Here's how the part is built. I have some questions about the finished solid (model axes, mm). Coordinates: 2 decimals unless noted, no trailing zeros. Write each loop counter-clockwise with the first axis right and the second up, starting at its lowest first coordinate (ties: lowest second). Pieces come first, ordered by that corner, then holes.
Item 1: If I drill on line 1 (X direction, y = -156, z = 2.75); line 2 (Y direction, x = -67.5, z = -1.75), over which ranges is the centre line in solid material (lowest first)?
Item 2: I'm going to push flat-ended pins straight in: pin 1 Ø10.5 at (x, y) = (-156, -156) entering from -Z; pin 2 Ø2.5 at (x, z) = (9, -1) entering from -Y; pin 3 Ø1.5 at (x, z) = (5, -1) entering from +Y; pin 4 Ø0.9 at (y, z) = (-1.5, -2) entering from +X. Where does each tip first touch, or does it pass through?
Item 3: We'd pull the mould along Y, two halves only. Please class faces 1 (the face through (-2, 2, 7)), 2 (the face through (-153.85, 159.373, 3.451)): +Y half, -Y half, draft (parallel to the pull), parting line (faces both ways), or undercut.
Item 4: If we section it at A-A (y = -156): Please give me the cut outline in (x, z), then the cut area to 3 significant figures.
Item 5: If we section it at C-C (y = 124): Please give me the cut outline in (x, z).
from build123d import *

# Parameters (mm, degrees)
F0_W     = 330
F0_H     = 330
F0_W_2   = 300
F0_H_2   = 300
F1_DEPTH = 7
F2_DEPTH = 3
F3_R     = 4
F4_DEPTH = 8


with BuildPart() as f1:
    # F0 (on Top) → F1 (new body)
    with BuildSketch(Plane.XY):
        Rectangle(F0_W, F0_H)
        Rectangle(F0_W_2, F0_H_2, mode=Mode.SUBTRACT)
        Rectangle(F0_W_2, F0_H_2)
    extrude(amount=F1_DEPTH)

    # F0 (on Top) → F2 (join)
    with BuildSketch(Plane.XY):
        Rectangle(F0_W_2, F0_H_2)
    extrude(amount=-F2_DEPTH)

    # F3 (on Top) → F4 (cut)
    with BuildSketch(Plane.XY):
        with Locations((-156, 156)):
            Circle(F3_R)
        with Locations((156, 156)):
            Circle(F3_R)
        with Locations((156, -156)):
            Circle(F3_R)
        with Locations((-156, -156)):
            Circle(F3_R)
    extrude(amount=F4_DEPTH, mode=Mode.SUBTRACT)


solid = f1.part
Answer list:
1. line 1: x = -165 to -160, -152 to 152, 160 to 165
1. line 2: y = -150 to 150
2. pin 1: stops at z = 0
2. pin 2: stops at y = -165
2. pin 3: stops at y = 150
2. pin 4: stops at x = 150
3. face 1: draft
3. face 2: undercut
4. outline: (-165, 0) - (-160, 0) - (-160, 7) - (-165, 7) - close; (-152, 0) - (152, 0) - (152, 7) - (-152, 7) - close; (160, 0) - (165, 0) - (165, 7) - (160, 7) - close
4. area: 2,200 mm2
5. outline: (-165, 0) - (-150, 0) - (-150, -3) - (150, -3) - (150, 0) - (165, 0) - (165, 7) - (-165, 7) - close
